from build123d import *

# Parameters (mm, degrees)
SKETCH_1_W          = 30
SKETCH_1_H          = 30
SKETCH_1_W_2        = 16.540501684
SKETCH_1_H_2        = 15
EXTRUDE_1_DEPTH     = 10
SKETCH_4_R          = 1.4
CUT_EXTRUDE_3_DEPTH = 24.452078799
SKETCH_8_R          = 2.9
CUT_EXTRUDE_6_DEPTH = 2
CHAMFER_1_SIZE      = 2
CHAMFER_1_SIZE_2    = 1.6
SKETCH_5_R          = 2.05
CUT_EXTRUDE_7_DEPTH = 20
SKETCH_9_R          = 2.8
SKETCH_9_R_2        = 2.2
CUT_EXTRUDE_8_DEPTH = 5
FILLET_1_R          = 1


with BuildPart() as part:
    # 스케치1 → 보스-돌출1 (new body)
    with BuildSketch(Plane(origin=(0, 0, 0), x_dir=(0, 0, -1), z_dir=(1, 0, 0))):
        Rectangle(SKETCH_1_W, SKETCH_1_H)
        Rectangle(SKETCH_1_W_2, SKETCH_1_H_2, mode=Mode.SUBTRACT)
    extrude(amount=EXTRUDE_1_DEPTH)

    # 스케치4 → 컷-돌출3 (cut, through all)
    with BuildSketch(Plane(origin=(0, 0, 0), x_dir=(0, 0, -1), z_dir=(1, 0, 0))):
        with Locations((-7, -12)):
            Circle(SKETCH_4_R)
        with Locations(Location((-7, 12, 0), (0, 0, 180))):
            Circle(SKETCH_4_R)
        with Locations(Location((7, -12, 0), (0, 0, 180))):
            Circle(SKETCH_4_R)
        with Locations((7, 12)):
            Circle(SKETCH_4_R)
    extrude(amount=CUT_EXTRUDE_3_DEPTH, mode=Mode.SUBTRACT)

    # 스케치8 → 컷-돌출6 (cut)
    with BuildSketch(Plane.ZY):
        with Locations((-7, 12)):
            Circle(SKETCH_8_R)
        with Locations((7, 12)):
            Circle(SKETCH_8_R)
        with Locations((-7, -12)):
            Circle(SKETCH_8_R)
        with Locations((7, -12)):
            Circle(SKETCH_8_R)
    extrude(amount=-CUT_EXTRUDE_6_DEPTH, mode=Mode.SUBTRACT)

    # 모따기1
    # the kernel refuses this chamfer: 2, 1.6 mm, written as the material it adds along each edge
    with BuildSketch(Plane(origin=(2, -12, 7), x_dir=(0, 0, 1), z_dir=(0, -1, 0))) as chamfer_1_piece_1_section:
        Polygon((2.9, CHAMFER_1_SIZE), (2.9 - CHAMFER_1_SIZE_2, 0), (2.9, 0), align=None)
    chamfer_1_piece_1 = revolve(axis=Axis((2, -12, 7), (-1, 0, 0)), mode=Mode.PRIVATE)
    chamfer_1_piece_1 = split(chamfer_1_piece_1, bisect_by=Plane(origin=(0, -12, 4.826759692), z_dir=(1, 0, 0)), keep=Keep.TOP, mode=Mode.PRIVATE)
    chamfer_1_piece_1 = chamfer_1_piece_1 - Plane(origin=(0.956092246, -12, 7), x_dir=(0, 0, -1), z_dir=(-1, 0, 0)) * Cylinder(1.4, 12, mode=Mode.PRIVATE)
    add(chamfer_1_piece_1)
    with BuildSketch(Plane(origin=(2, 12, 7), x_dir=(0, 0, 1), z_dir=(0, -1, 0))) as chamfer_1_piece_2_section:
        Polygon((2.9, CHAMFER_1_SIZE), (2.9 - CHAMFER_1_SIZE_2, 0), (2.9, 0), align=None)
    chamfer_1_piece_2 = revolve(axis=Axis((2, 12, 7), (-1, 0, 0)), mode=Mode.PRIVATE)
    chamfer_1_piece_2 = split(chamfer_1_piece_2, bisect_by=Plane(origin=(0, 12, 4.826759692), z_dir=(1, 0, 0)), keep=Keep.TOP, mode=Mode.PRIVATE)
    chamfer_1_piece_2 = chamfer_1_piece_2 - Plane(origin=(0.956092246, 12, 7), x_dir=(0, 0, 1), z_dir=(-1, 0, 0)) * Cylinder(1.4, 12, mode=Mode.PRIVATE)
    add(chamfer_1_piece_2)
    with BuildSketch(Plane(origin=(2, 12, -7), x_dir=(0, 0, 1), z_dir=(0, -1, 0))) as chamfer_1_piece_3_section:
        Polygon((2.9, CHAMFER_1_SIZE), (2.9 - CHAMFER_1_SIZE_2, 0), (2.9, 0), align=None)
    chamfer_1_piece_3 = revolve(axis=Axis((2, 12, -7), (-1, 0, 0)), mode=Mode.PRIVATE)
    chamfer_1_piece_3 = split(chamfer_1_piece_3, bisect_by=Plane(origin=(0, 12, -9.173240308), z_dir=(1, 0, 0)), keep=Keep.TOP, mode=Mode.PRIVATE)
    chamfer_1_piece_3 = chamfer_1_piece_3 - Plane(origin=(0.956092246, 12, -7), x_dir=(0, 0, -1), z_dir=(-1, 0, 0)) * Cylinder(1.4, 12, mode=Mode.PRIVATE)
    add(chamfer_1_piece_3)
    with BuildSketch(Plane(origin=(2, -12, -7), x_dir=(0, 0, 1), z_dir=(0, -1, 0))) as chamfer_1_piece_4_section:
        Polygon((2.9, CHAMFER_1_SIZE), (2.9 - CHAMFER_1_SIZE_2, 0), (2.9, 0), align=None)
    chamfer_1_piece_4 = revolve(axis=Axis((2, -12, -7), (-1, 0, 0)), mode=Mode.PRIVATE)
    chamfer_1_piece_4 = split(chamfer_1_piece_4, bisect_by=Plane(origin=(0, -12, -9.173240308), z_dir=(1, 0, 0)), keep=Keep.TOP, mode=Mode.PRIVATE)
    chamfer_1_piece_4 = chamfer_1_piece_4 - Plane(origin=(0.956092246, -12, -7), x_dir=(0, 0, 1), z_dir=(-1, 0, 0)) * Cylinder(1.4, 12, mode=Mode.PRIVATE)
    add(chamfer_1_piece_4)

    # 스케치5 → 컷-돌출7 (cut)
    with BuildSketch(Plane(origin=(0, 0, 0), x_dir=(1, 0, 0), z_dir=(0, 1, 0))):
        with Locations(Location((5, 0, 0), (0, 0, 270))):
            Circle(SKETCH_5_R)
    extrude(amount=-CUT_EXTRUDE_7_DEPTH, mode=Mode.SUBTRACT)

    # 스케치9 → 컷-돌출8 (cut)
    with BuildSketch(Plane.XZ.offset(-7.5)):
        with Locations(Location((5, 0, 0), (0, 0, 270))):
            Circle(SKETCH_9_R)
        with Locations(Location((5, 0, 0), (0, 0, 270))):
            Circle(SKETCH_9_R_2, mode=Mode.SUBTRACT)
    extrude(amount=-CUT_EXTRUDE_8_DEPTH, mode=Mode.SUBTRACT)

    # 필렛1
    fillet_1_edges = [part.edges().sort_by_distance(p)[0] for p in [
        (5, 7.5, 2.2),
    ]]
    fillet(fillet_1_edges, radius=FILLET_1_R)


solid = part.part
Can you work these out from the model? Positions are in its coordinate system, mm. A direction names the side the tool comes from. Give positions to 0.01 mm unless a question says otherwise; leave off trailing zeros. Order: outer loops, then holes, each group sorted by start corner. A loop starts at its lowest first (then second) coordinate and runs counter-clockwise, first axis right, second up. Notation, with made-up numbers: M 43,-12.5 L 80,-12.5 A18 cw 80,22.5 Z; hole C 86,-12.5 d9. An arc over 180 degrees is marked long. Use one line per item in the form item = value. Start each with the question number.
Item 1: If we section it at D-D (x = 9): Write out the boundary of the cut face in (y, z), then the cut area to 3 significant figures.
Item 2: If we section it at A-A (y = -12): Write out the boundary of the cut face in (x, z) (3 decimals), then the cut area to 3 significant figures.
Item 3: If I drill on line 1 along Y through (x, z) = (8, -7); line 2 along Z through (x, y) = (7.25, -12); line 3 along Z through (x, y) = (5.5, 12) (3 decimals), over which ranges is the centre line in solid material (lowest first)?
Item 4: Will this pin go through, and if not, where does the flat tip stop? pin 1 Ø2.5 at (x, z) = (5, 0) entering from -Y.
Item 5: If we section it at B-B (y = 12): Write out the boundary of the cut face in (x, z) (3 decimals), then the cut area to 3 significant figures.
Item 6: We'd pull the mould along Y, two halves only. Please class faces 1 (the cylindrical face through (5.88, -11.05, -8.03)), 2 (the flat face through (5, 15, 0)), 3 (the flat face through (5, 0, 15)): +Y half, -Y half, draft (parallel to the pull), parting line (faces both ways), or undercut.
Item 7: If we section it at C-C (z = 3.5): Write out the boundary of the cut face in (x, y).
Item 8: For faces 4 (the flat face through (4, -7.5, 2)), 5 (the cylindrical face through (7.18, 10.47, 0.29)), 6 (the flat face through (5, 0, -15)), which set-ups out of +Z, -Z, +X, -X, +Y, -Y let a thin tool reach every point of the face, with its end or its side?
Outcome:
q1.outline = M -15,-15 L 15,-15 L 15,15 L -15,15 Z; hole C -12,-7 d2.8; hole C -12,7 d2.8; hole M -7.5,-8.27 L 7.5,-8.27 L 7.5,8.27 L -7.5,8.27 Z; hole C 12,-7 d2.8; hole C 12,7 d2.8
q1.area = 627 mm2
q2.outline = M 0,-15 L 10,-15 L 10,-8.4 L 1.875,-8.4 L 0,-9.9 Z; M 0,-4.1 L 1.875,-5.6 L 10,-5.6 L 10,5.6 L 1.875,5.6 L 0,4.1 Z; M 0,9.9 L 1.875,8.4 L 10,8.4 L 10,15 L 0,15 Z; hole C 5,0 d4.1
q2.area = 225 mm2
q3.line_1 = -15 to -13.4, -10.6 to -7.5, 7.5 to 10.6, 13.4 to 15
q3.line_2 = -15 to -8.4, -5.6 to 5.6, 8.4 to 15
q3.line_3 = -15 to -8.4, -5.6 to -2.755, -2.142 to 2.142, 2.755 to 5.6, 8.4 to 15
q4.pin_1 = 7.5
q5.outline = M 0,-15 L 10,-15 L 10,-8.4 L 1.875,-8.4 L 0,-9.9 Z; M 0,-4.1 L 1.875,-5.6 L 10,-5.6 L 10,5.6 L 1.875,5.6 L 0,4.1 Z; M 0,9.9 L 1.875,8.4 L 10,8.4 L 10,15 L 0,15 Z; C 5,0 d4.4; hole C 5,0 d5.6
q5.area = 229 mm2
q6.face_1 = undercut
q6.face_2 = +Y half
q6.face_3 = draft
q7.outline = M 0,-15 L 10,-15 L 10,-7.5 L 0,-7.5 Z; M 0,7.5 L 10,7.5 L 10,15 L 0,15 Z
q8.face_4 = +X, -X
q8.face_5 = none
q8.face_6 = -Z, +X, -X, +Y, -Y
